from build123d import *

# Parameters (mm, degrees)
BOSS_EXTRUDE1_DEPTH = 1.5875


with BuildPart() as part:
    # Sketch1 → Boss-Extrude1 (new body)
    with BuildSketch(Plane.XY):
        Polygon((6453.274222112, 2700.300995821), (6453.274222112, 2697.125995821), (6446.467022112, 2697.125995821), (6446.467022112, 2687.931195821), (6767.942122112, 2687.931195821), (6767.942122112, 2694.116095821), (6793.342122112, 2694.116095821), (6793.342122112, 2700.300995821), (6749.901772112, 2700.300995821), (6749.901772112, 2697.125995821), (6746.498172112, 2697.125995821), (6746.498172112, 2700.300995821), (6681.842472112, 2700.300995821), (6681.842472112, 2697.125995821), (6678.438872112, 2697.125995821), (6678.438872112, 2700.300995821), (6616.958172112, 2700.300995821), (6616.958172112, 2697.125995821), (6613.554572112, 2697.125995821), (6613.554572112, 2700.300995821), (6548.898872112, 2700.300995821), (6548.898872112, 2697.125995821), (6545.495272112, 2697.125995821), (6545.495272112, 2700.300995821), (6484.014572112, 2700.300995821), (6484.014572112, 2697.125995821), (6480.839572112, 2697.125995821), (6480.839572112, 2700.300995821), align=None)
        Polygon((6484.260159217, 2689.353595821), (6486.093246321, 2692.528595821), (6484.260159217, 2695.703595821), (6480.593985007, 2695.703595821), (6478.760897903, 2692.528595821), (6480.593985007, 2689.353595821), align=None, mode=Mode.SUBTRACT)
        Polygon((6549.144459217, 2689.353595821), (6550.977546321, 2692.528595821), (6549.144459217, 2695.703595821), (6545.478285007, 2695.703595821), (6543.645197903, 2692.528595821), (6545.478285007, 2689.353595821), align=None, mode=Mode.SUBTRACT)
        Polygon((6617.203759217, 2689.353595821), (6619.036846321, 2692.528595821), (6617.203759217, 2695.703595821), (6613.537585007, 2695.703595821), (6611.704497903, 2692.528595821), (6613.537585007, 2689.353595821), align=None, mode=Mode.SUBTRACT)
        Polygon((6682.088059217, 2689.353595821), (6683.921146321, 2692.528595821), (6682.088059217, 2695.703595821), (6678.421885007, 2695.703595821), (6676.588797903, 2692.528595821), (6678.421885007, 2689.353595821), align=None, mode=Mode.SUBTRACT)
        Polygon((6750.147359217, 2689.353595821), (6751.980446321, 2692.528595821), (6750.147359217, 2695.703595821), (6746.481185007, 2695.703595821), (6744.648097903, 2692.528595821), (6746.481185007, 2689.353595821), align=None, mode=Mode.SUBTRACT)
        Polygon((6453.519809217, 2689.353595821), (6455.352896321, 2692.528595821), (6453.519809217, 2695.703595821), (6449.853635007, 2695.703595821), (6448.020547903, 2692.528595821), (6449.853635007, 2689.353595821), align=None, mode=Mode.SUBTRACT)
    extrude(amount=BOSS_EXTRUDE1_DEPTH)


solid = part.part
Geometry check sheet. Reference: the model listing, model coordinates, mm. Give positions to 0.01 mm unless a question says otherwise; leave off trailing zeros. Answer as a JSON object with one key per item and string values. Group by question number.
Item 1: Sectioned sample at A-A on z = 1.05. Give the number of separate pieces and of enclosed holes in the cut face, plus the area to 3 significant figures.
Item 2: Material ranges on L1, parallel to X at y = 2697.25, z = 0.2; L2, parallel to X at y = 2688.75, z = 1.5, recorded low to high.
Item 3: Gauge pin test, flat end, axial feed: pin 1 (0.5 mm diameter, centred on x = 6482.5, z = 1, fed in from +Y). Record the tip position at first contact, or that the pin passes through.
Findings below:
{
 "1": {"separate pieces": "1", "enclosed holes": "6", "area": "3,850 mm2"},
 "2": {"L1": "6453.27 to 6480.84, 6484.01 to 6545.5, 6548.9 to 6613.55, 6616.96 to 6678.44, 6681.84 to 6746.5, 6749.9 to 6793.34", "L2": "6446.47 to 6767.94"},
 "3": {"pin 1": "y = 2697.13"}
}
